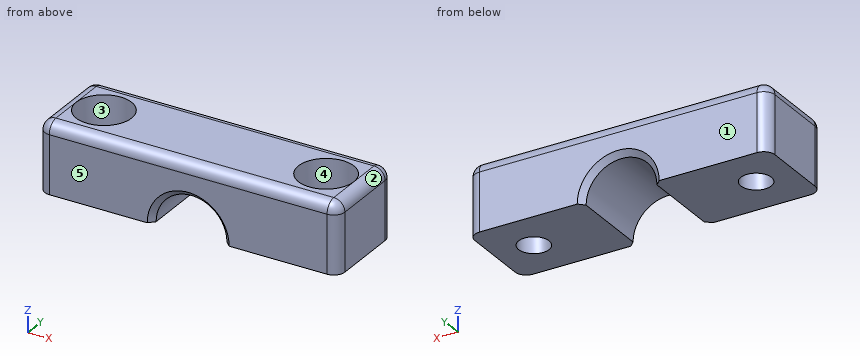
from build123d import *

# Parameters (mm, degrees)
F1_DEPTH = 16
F3_DEPTH = 12.501
F4_R     = 5
F4_R_2   = 2.75
F5_DEPTH = 6
F6_SIZE  = 1
F7_R     = 2
F8_R     = 1.99999


# Not quite as in the source:
# - a fillet or chamfer is up to 0.001 mm smaller than in the source, because OpenCascade refuses the exact size


with BuildPart() as f1:
    # F0 (on Front) → F1 (new body)
    with BuildSketch(Plane.XZ):
        with BuildLine():
            Line((27, 12.5), (-27, 12.5))
            Line((-27, 12.5), (-27, 0))
            Line((-27, 0), (-6.375, 0))
            ThreePointArc((-6.375, 0), (0, 6.375), (6.375, 0))
            Line((6.375, 0), (27, 0))
            Line((27, 0), (27, 12.5))
        make_face()
    extrude(amount=F1_DEPTH)

    # F2 (on face) → F3 (cut, through all)
    with BuildSketch(Plane.XY.offset(12.5)):
        with BuildLine():
            Line((-22.75, -8), (-17.25, -8))
            ThreePointArc((-17.25, -8), (-20, -5.25), (-22.75, -8))
        make_face()
        with BuildLine():
            ThreePointArc((-22.75, -8), (-20, -10.75), (-17.25, -8))
            Line((-17.25, -8), (-22.75, -8))
        make_face()
        with BuildLine():
            Line((17.25, -8), (22.75, -8))
            ThreePointArc((22.75, -8), (20, -5.25), (17.25, -8))
        make_face()
        with BuildLine():
            ThreePointArc((17.25, -8), (20, -10.75), (22.75, -8))
            Line((22.75, -8), (17.25, -8))
        make_face()
    extrude(amount=-F3_DEPTH, mode=Mode.SUBTRACT)

    # F4 (on face) → F5 (cut)
    with BuildSketch(Plane.XY.offset(12.5)):
        with Locations((-20, -8)):
            Circle(F4_R)
        with Locations((-20, -8)):
            Circle(F4_R_2, mode=Mode.SUBTRACT)
        with Locations((20, -8)):
            Circle(F4_R)
        with Locations((20, -8)):
            Circle(F4_R_2, mode=Mode.SUBTRACT)
    extrude(amount=-F5_DEPTH, mode=Mode.SUBTRACT)

    # F6
    f6_edges = [f1.edges().sort_by_distance(p)[0] for p in [
        (0, -16, 6.375),
        (0, 0, 6.375),
    ]]
    chamfer(f6_edges, length=F6_SIZE)

    # F7
    f7_edges = [f1.edges().sort_by_distance(p)[0] for p in [
        (27, 0, 6.25),
        (27, -16, 6.25),
        (-27, 0, 6.25),
        (-27, -16, 6.25),
    ]]
    fillet(f7_edges, radius=F7_R)

    # F8 (radius 2 in the source; OpenCascade refuses exactly that, so slightly less here)
    f8_edges = [f1.edges().sort_by_distance(p)[0] for p in [
        (0, 0, 12.5),
    ]]
    fillet(f8_edges, radius=F8_R)


solid = f1.part
Read the model definition and answer for the solid it produces. Units are mm, in the model's axes. Face numbers are marked on the shaded views. A direction names the side the tool comes from. Give positions to 0.01 mm unless a question says otherwise; leave off trailing zeros. Write each loop counter-clockwise with the first axis right and the second up, starting at its lowest first coordinate (ties: lowest second). Pieces come first, ordered by that corner, then holes. Notation, with made-up numbers: (39.25, 86) - (70.25, 86) arc R16 ccw to (70.25, 94) - close; hole circle Ø9 at (-33, 16). An arc over 180 degrees is marked (long way). Use CSV: the item, a comma, the result in double quotes. Start each with the question number.
(1) Find section A-A (y = -8). Count the separate pieces of the cut face and the enclosed holes in it, plus the area to 3 significant figures.
(2) Consider line 1 along X through (y, z) = (-9.5, 8.5); line 2 along X through (y, z) = (-8, 5.25); line 3 along Y through (x, z) = (-20, 1.5). Determine where each line is inside the solid, lowest interval first.
(3) Find section B-B (x = -20). Give the vertices of the cut face in (y, z).
(4) For the marked faces 4 and 5, determine the directions among +Z, -Z, +X, -X, +Y, -Y from which every point of the face is accessible in a straight line to the end or side of a thin tool.
(5) Find section C-C (z = 9.5). Give the vertices of the cut face in (x, y).
(6) Given P1, Ø9, axis at x = 20, y = -8, coming from the +Z side, flat-ended and moving along its own axis, determine where the tip first touches the part or whether it passes through.
(7) Determine the mould class of the marked faces 1, 2 and 3 for opening direction Y: +Y half, -Y half, draft (parallel to the pull), parting line (faces both ways), or undercut.
(8) Find section D-D (x = 0). Give the vertices of the cut face in (y, z) (3 decimals), plus the area to 3 significant figures.
Findings below:
1,separate pieces,"3"
1,enclosed holes,"0"
1,area,"418 mm2"
2,line 1,"-27 to -24.77, -15.23 to 15.23, 24.77 to 27"
2,line 2,"-27 to -22.75, -17.25 to -3.62, 3.62 to 17.25, 22.75 to 27"
2,line 3,"-16 to -10.75, -5.25 to 0"
3,outline,"(-16, 0) - (-10.75, 0) - (-10.75, 6.5) - (-13, 6.5) - (-13, 12.5) - (-14, 12.5) arc R2 ccw to (-16, 10.5) - close; (-5.25, 0) - (0, 0) - (0, 10.5) arc R2 ccw to (-2, 12.5) - (-3, 12.5) - (-3, 6.5) - (-5.25, 6.5) - close"
4,face 4,"+Z"
4,face 5,"+Z, -Z, +X, -X, -Y"
5,outline,"(-27, -14) arc R2 ccw to (-25, -16) - (25, -16) arc R2 ccw to (27, -14) - (27, -2) arc R2 ccw to (25, 0) - (-25, 0) arc R2 ccw to (-27, -2) - close; hole circle Ø10 at (-20, -8); hole circle Ø10 at (20, -8)"
6,P1,"z = 6.5"
7,face 1,"+Y half"
7,face 2,"draft"
7,face 3,"undercut"
8,outline,"(-16, 7.375) - (-15, 6.375) - (-1, 6.375) - (0, 7.375) - (0, 10.5) arc R2 ccw to (-2, 12.5) - (-14, 12.5) arc R2 ccw to (-16, 10.5) - close"
8,area,"95.3 mm2"
